Autodesk Inventor part; units mm, degrees
ref_plane "YZ Plane" through (0, 0, 0) normal (1, 0, 0) x (0, 1, 0)
ref_plane "XZ Plane" through (0, 0, 0) normal (0, 1, 0) x (-1, 0, 0)
ref_plane "XY Plane" through (0, 0, 0) normal (0, 0, 1) x (1, 0, 0)
sketch "Sketch1" plane through (0, 0, 0) normal (0, 0, 1) x (1, 0, 0)
  line L0 (0, -42.5799) -> (0, 42.5799)
  line L1 (-42.5799, 0) -> (42.5799, 0)
  line L2 (-28, 30) -> (28, 30)
  line L3 (30, 28) -> (30, -28)
  line L4 (28, -30) -> (-28, -30)
  line L5 (-30, -28) -> (-30, 28)
  arc A0 (-28, 30) -> (-30, 28) centre (-28, 28) ccw
  arc A1 (30, 28) -> (28, 30) centre (28, 28) ccw
  arc A2 (28, -30) -> (30, -28) centre (28, -28) ccw
  arc A3 (-30, -28) -> (-28, -30) centre (-28, -28) ccw
  point P0 (0, 0)
  point P1 (-30, 30)
  point P2 (30, 30)
  point P3 (-22.4506, 22.4506)
  point P4 (-26.5, 15)
  point P5 (-15, 26.5)
  point P6 (-15, -26.5)
  point P7 (-22.4506, -22.4506)
  point P8 (-26.5, -15)
  point P9 (26.5, -15)
  point P10 (22.4506, -22.4506)
  point P11 (15, -26.5)
  point P12 (15, 26.5)
  point P13 (22.4506, 22.4506)
  point P14 (26.5, 15)
  dimension "d0" = 60
  dimension "d1" = 2
  dimension "d2" = 22.4506
  dimension "d3" = 22.4506
  dimension "d4" = 15
  dimension "d5" = 15
  dimension "d6" = 3.5
  dimension "d7" = 3.5
  dimension "d10" = 360
extrude "Extrusion1" add sketch "Sketch1" against normal blind 2
hole "Hole1" at (-22.4506, 22.4506, 0) at (22.4506, 22.4506, 0) at (22.4506, -22.4506, 0) at (-22.4506, -22.4506, 0) direction (0, 0, -1) diameter 3.4 end through all
hole "Hole2" at (-26.5, 15, 0) at (-15, 26.5, 0) at (-15, -26.5, 0) at (-26.5, -15, 0) at (26.5, -15, 0) at (15, -26.5, 0) at (15, 26.5, 0) at (26.5, 15, 0) direction (0, 0, -1) diameter 2.4 end through all
equation "\"d12\" = front_plate_thickness"
equation "\"encoder_axis\" = 8"
equation "\"encoder_emboss\" = 0"
equation "\"encoders\" = 0"
equation "\"encoder_width\" = 27"
equation "\"front_plate_thickness\" = 2"
equation "\"glass_thickness\" = 2"
equation "\"screw_distance_outside\" = 3.5"
equation "\"encoder_rad\" = 49"
equation "\"encoder_extrude_hight\" = 3"
equation "\"screw_distance_center\" = 15"
equation "\"ring_top_thickness\" = 2"
equation "\"ring_outer_bevel_depth\" = 0.5"
equation "\"ring_depth\" = 6"
equation "\"ring_outer_bevel_height\" = 3"
equation "\"ring_inner_bevel_depth\" = 3.5"
equation "\"ring_thickness\" = 9"
equation "\"hole_from_center\" = 63.5"
equation "\"circle_dimension_inner\" = 47"
equation "\"circle_dimension\" = 56"
equation "\"backplate_width\" = 60"
equation "\"hole_distance\" = 22.45064"
properties part number "FrontGlass" material "Polycarbonate, Clear"
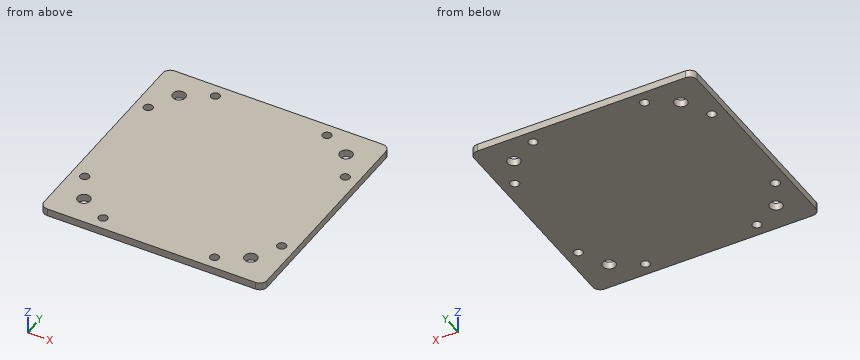
Input: part model. Units: mm. Frame: model coordinates. Round coordinates to 2 decimals unless told otherwise and drop trailing zeros. Write each loop counter-clockwise with the first axis right and the second up, starting at its lowest first coordinate (ties: lowest second). Pieces come first, ordered by that corner, then holes.
1) Cut plane A-A (x = 26.5). Return the cut outline in (y, z).
2) Ray query, L1, parallel to X at y = 15, z = -1.3; L2, parallel to Y at x = -26.5, z = -1.25. Return the intervals inside material, ascending.
3) Cut plane C-C (z = -0.55). Count the separate pieces of the cut face and the enclosed holes in it, then the cut area to 3 significant figures.
Geometry says:
1. outline: (-30, -2) - (-16.2, -2) - (-16.2, 0) - (-30, 0) - close; (-13.8, -2) - (13.8, -2) - (13.8, 0) - (-13.8, 0) - close; (16.2, -2) - (30, -2) - (30, 0) - (16.2, 0) - close
2. L1: x = -30 to -27.7, -25.3 to 25.3, 27.7 to 30
2. L2: y = -30 to -16.2, -13.8 to 13.8, 16.2 to 30
3. separate pieces: 1
3. enclosed holes: 12
3. area: 3,520 mm2
